Geometry: see drawing. Coordinates: mm, zero at the bounding-box minimum. Round coordinates to 2 decimals unless told otherwise and drop trailing zeros. Loops run counter-clockwise (first coordinate to the right, second up) from the corner with the lowest first, then second, coordinate; pieces in that order, holes last.
(1) Cut plane A-A, the plane z = 11.55. Output: boundary loops of the cut face in (x, y).
(2) Cut plane D-D, the plane y = 0.8. Give the number of separate pieces and of enclosed holes in the cut face, and give its area (3 significant figures).
(3) Cut plane C-C, the plane x = 34.68. Output: boundary loops of the cut face in (y, z).
(4) Line query: line 1 (X direction, y = 0.85, z = 11.55); line 2 (X direction, y = 0.5, z = 14.5); line 3 (Z direction, x = 29.5, y = 0.5). Output: solid intervals per line, ascending.
(5) Cut plane B-B, the plane z = 21.71. Output: boundary loops of the cut face in (x, y).
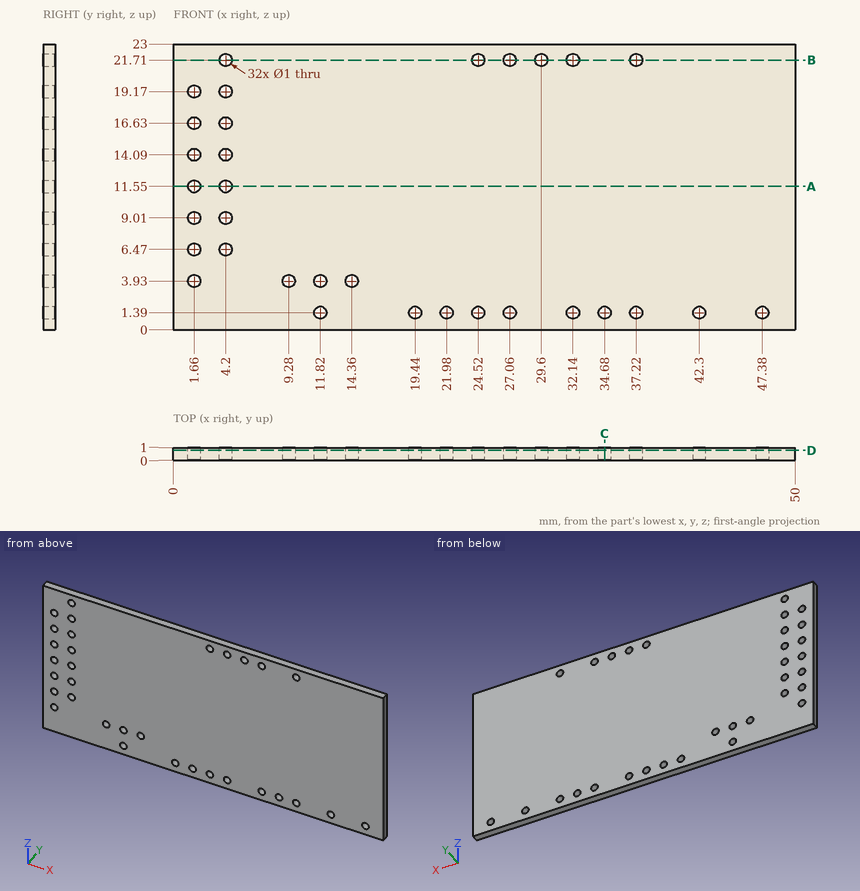
Reported:
1. outline: (0, 0) - (1.16, 0) - (1.16, 1) - (0, 1) - close; (2.16, 0) - (3.7, 0) - (3.7, 1) - (2.16, 1) - close; (4.7, 0) - (50, 0) - (50, 1) - (4.7, 1) - close
2. separate pieces: 1
2. enclosed holes: 32
2. area: 1,120 mm2
3. outline: (0, 0) - (1, 0) - (1, 0.89) - (0, 0.89) - close; (0, 1.89) - (1, 1.89) - (1, 23) - (0, 23) - close
4. line 1: x = 0 to 1.16, 2.16 to 3.7, 4.7 to 50
4. line 2: x = 0 to 1.37, 1.95 to 3.91, 4.49 to 50
4. line 3: z = 0 to 21.22, 22.2 to 23
5. outline: (0, 0) - (3.7, 0) - (3.7, 1) - (0, 1) - close; (4.7, 0) - (24.02, 0) - (24.02, 1) - (4.7, 1) - close; (25.02, 0) - (26.56, 0) - (26.56, 1) - (25.02, 1) - close; (27.56, 0) - (29.1, 0) - (29.1, 1) - (27.56, 1) - close; (30.1, 0) - (31.64, 0) - (31.64, 1) - (30.1, 1) - close; (32.64, 0) - (36.72, 0) - (36.72, 1) - (32.64, 1) - close; (37.72, 0) - (50, 0) - (50, 1) - (37.72, 1) - close
